Autodesk Inventor part; units mm, degrees
ref_plane "YZ Plane" through (0, 0, 0) normal (1, 0, 0) x (0, 1, 0)
ref_plane "XZ Plane" through (0, 0, 0) normal (0, 1, 0) x (-1, 0, 0)
ref_plane "XY Plane" through (0, 0, 0) normal (0, 0, 1) x (1, 0, 0)
sketch "Sketch1" plane through (0, 0, 0) normal (0, 0, 1) x (1, 0, 0)
  arc A0 (14.2748, -15.875) -> (15.875, -14.2748) centre (14.2748, -14.2748) ccw
  line L0 (15.875, -14.2748) -> (15.875, 14.2748)
  line L1 (14.2748, 15.875) -> (-14.2748, 15.875)
  arc A1 (-14.2748, 15.875) -> (-15.875, 14.2748) centre (-14.2748, 14.2748) ccw
  line L2 (-15.875, 14.2748) -> (-15.875, -14.2748)
  arc A2 (-15.875, -14.2748) -> (-14.2748, -15.875) centre (-14.2748, -14.2748) ccw
  line L3 (-14.2748, -15.875) -> (14.2748, -15.875)
  arc A3 (15.875, 14.2748) -> (14.2748, 15.875) centre (14.2748, 14.2748) ccw
  line L4 (-15.875, -19.05) -> (56.769, -19.05)
  line L5 (56.769, -19.05) -> (57.15, -18.669)
  line L6 (57.15, -18.669) -> (57.15, -16.256)
  line L7 (57.15, -16.256) -> (56.769, -15.875)
  line L8 (56.769, -15.875) -> (20.6502, -15.875)
  arc A4 (19.05, -14.2748) -> (20.6502, -15.875) centre (20.6502, -14.2748) ccw
  line L9 (19.05, -14.2748) -> (19.05, 14.2748)
  arc A5 (20.6502, 15.875) -> (19.05, 14.2748) centre (20.6502, 14.2748) ccw
  line L10 (20.6502, 15.875) -> (56.769, 15.875)
  line L11 (56.769, 15.875) -> (57.15, 16.256)
  line L12 (57.15, 16.256) -> (57.15, 18.669)
  line L13 (57.15, 18.669) -> (56.769, 19.05)
  line L14 (56.769, 19.05) -> (-15.875, 19.05)
  arc A6 (-15.875, 19.05) -> (-19.05, 15.875) centre (-15.875, 15.875) ccw
  line L15 (-19.05, 15.875) -> (-19.05, -15.875)
  arc A7 (-19.05, -15.875) -> (-15.875, -19.05) centre (-15.875, -15.875) ccw
  point P0 (0, 0)
extrude "Extrusion1" add sketch "Sketch1" against normal blind 304.8
hole "Hole1" at (-19.05, 0, -19.05) direction (1, 0, 0) diameter 8.3312 end through all
hole "Hole2" at (0, 19.05, -19.05) direction (0, -1, 0) diameter 8.3312 end through all
pattern_linear "Rectangular Pattern1" count 200 spacing 38.1 along (0, 0, -1) of "Hole2", "Hole1"
properties part number "9726"
Geometry check sheet. Reference: the model listing, model coordinates, mm. A direction names the side the tool comes from. Coordinates: 2 decimals unless noted, no trailing zeros. Write each loop counter-clockwise with the first axis right and the second up, starting at its lowest first coordinate (ties: lowest second). Pieces come first, ordered by that corner, then holes. Notation, with made-up numbers: M 83.25,65.5 L 135.25,65.5 A29 ccw 135.25,101.5 Z; hole C 81,16.5 d8. An arc over 180 degrees is marked long. One line per item, written item: value. Start each with the question number.
(1) Tool access check on faces 1 (the face through (15.875, 0, -150)), 2 (the face through (-17.44, -2.815, -60.22)), 3 (the face through (39, -15.875, -150)). Record the directions out of +Z, -Z, +X, -X, +Y, -Y that give a thin tool (end or side, any length) a straight path to the whole face; none if there is none.
(2) Release check for a two-part mould opening along Z. For faces 4 (the face through (21, 19.05, -150)), 5 (the face through (17.485, -2.815, -22.12)) record: released by +Z, released by -Z, zero draft, split by the parting line, or undercut.
(3) Sectioned sample at B-B, the plane x = -8. Enter the section's corners in (y, z) (3 decimals).
(4) Scan lines: line 1 along X through (y, z) = (-11.5, -235) (3 decimals); line 2 along Y through (x, z) = (16.7, -57.15). Record each from-to range of solid material in increasing order. Write a range as [from, to].
(5) Sectioned sample at C-C, the plane z = -57.15. State how many separate pieces and enclosed holes the cut face has, and give its area (3 significant figures).
(6) Sectioned sample at A-A, the plane z = -186.5. Enter the section's corners in (x, y) (3 decimals).
(7) Depth check by flat-ended pin: pin 1 (6.5 mm diameter, centred on y = 0, z = -95.25, fed in from +X); pin 2 (13.5 mm diameter, centred on y = 0, z = -247.65, fed in from +X). Enter the tip coordinate at first touch or a pass-through.
Filled sheet:
1. face 1: +Z, -Z
1. face 2: +X, -X
1. face 3: +Z, -Z, +X
2. face 4: zero draft
2. face 5: undercut
3. outline: M -19.05,-304.8 L -15.875,-304.8 L -15.875,0 L -19.05,0 Z; M 15.875,-304.8 L 19.05,-304.8 L 19.05,0 L 15.875,0 Z
4. line 1: [-19.05, -15.875], [15.875, 19.05]
4. line 2: [-19.05, -4.17], [4.17, 19.05]
5. separate pieces: 4
5. enclosed holes: 0
5. area: 578 mm²
6. outline: M -19.05,-15.875 A3.175 ccw -15.875,-19.05 L 56.769,-19.05 L 57.15,-18.669 L 57.15,-16.256 L 56.769,-15.875 L 20.65,-15.875 A1.6 cw 19.05,-14.275 L 19.05,14.275 A1.6 cw 20.65,15.875 L 56.769,15.875 L 57.15,16.256 L 57.15,18.669 L 56.769,19.05 L -15.875,19.05 A3.175 ccw -19.05,15.875 Z; hole M -15.875,-14.275 A1.6 ccw -14.275,-15.875 L 14.275,-15.875 A1.6 ccw 15.875,-14.275 L 15.875,14.275 A1.6 ccw 14.275,15.875 L -14.275,15.875 A1.6 ccw -15.875,14.275 Z
7. pin 1: through
7. pin 2: x = 19.05
